CAD build for the part. Positions are in the model's coordinates, mm. Round coordinates to 2 decimals unless told otherwise and drop trailing zeros. Write each loop counter-clockwise with the first axis right and the second up, starting at its lowest first coordinate (ties: lowest second). Pieces come first, ordered by that corner, then holes. Notation, with made-up numbers: (-32.75, -35) - (-11.75, -35) arc R10 cw to (-11.75, -28) - close; hole circle Ø6 at (79, 42.25). An arc over 180 degrees is marked (long way). Put each result on its own line as item: value. Start each with the question number.
Item 1: Mould opens along X. For faces 1 (the flat face through (1, 6, 3)), 2 (the flat face through (4, 6, 1)), 3 (the cylindrical face through (2, 4.3, 1.5)), 4 (the flat face through (-2.5, 6, 1)) say: released by +X, released by -X, zero draft, split by the parting line, or undercut.
Item 2: Drill centre lines: line 1 (Y direction, x = 2, z = 1.75) (3 decimals); line 2 (X direction, y = 10.7, z = 0.8) (3 decimals); line 3 (Y direction, x = 1.75, z = 0.9). Where is each one in solid material? Low to high. Write a range as from..to.
Item 3: Cut at C-C (z = 1.8). Give the cut face in (x, y) (3 decimals).
Item 4: Cut at A-A (x = 2). Give the cut face in (y, z) (3 decimals).
Item 5: Cut at B-B (y = 1.3). Give the cut face in (x, z) (3 decimals), and give its area (3 significant figures).
Item 6: Cut at D-D (y = 3.5). Give the cut face in (x, z), and give its area (3 significant figures).
Autodesk Inventor part; units mm, degrees
ref_plane "YZ Plane" through (0, 0, 0) normal (1, 0, 0) x (0, 1, 0)
ref_plane "XZ Plane" through (0, 0, 0) normal (0, 1, 0) x (-1, 0, 0)
ref_plane "XY Plane" through (0, 0, 0) normal (0, 0, 1) x (1, 0, 0)
sketch "스케치1" plane through (0, 0, 0) normal (0, 0, 1) x (1, 0, 0)
  line L0 (0, 0) -> (4, 0)
  line L1 (4, 0) -> (4, 12)
  line L2 (4, 12) -> (0, 12)
  line L3 (0, 12) -> (0, 0)
  dimension "d0" = 4
  dimension "d1" = 12
extrude "돌출1" add sketch "스케치1" along normal blind 3
sketch "스케치2" plane through (0, 0, 3) normal (0, 0, 1) x (1, 0, 0)
  line L0 (4, 12) -> (0, 12) construction
  line L1 (2, 12) -> (2, 0) construction
  line L2 (0, 0) -> (4, 0) construction
  line L3 (4, 0) -> (4, 12)
  line L4 (0, 12) -> (0, 0)
  point P0 (2, 7.7)
  point P1 (2, 3.5)
  point P2 (2, 1.3)
  point P3 (2, 10.7)
  dimension "d9" = 4.3
  dimension "d45" = 1.3
  dimension "d51" = 4.2
  dimension "d52" = 2.2
  dimension "d55" = 1.3
hole "구멍2" at (2, 3.5, 3) direction (0, 0, -1) diameter 1.6 end through all
hole "구멍3" at (2, 1.3, 3) at (2, 10.7, 3) direction (0, 0, -1) diameter 0.63 end through all
sketch "스케치4" plane through (0, 0, 0) normal (-1, 0, 0) x (0, 0, 1)
  line L0 (0, 12) -> (0, 0)
  line L1 (0, 0) -> (3, 0)
  line L2 (3, 12) -> (3, 0)
  line L3 (0, 12) -> (3, 12)
extrude "돌출4" add sketch "스케치4" along normal blind 2.5
equation "\"G23_M\" = 0.67"
equation "\"G23_F\" = 0.65"
properties part number "_3D 인쇄"
Output values:
1. face 1: zero draft
1. face 2: released by +X
1. face 3: undercut
1. face 4: released by -X
2. line 1: 0..0.985, 1.615..2.7, 4.3..10.385, 11.015..12
2. line 2: -2.5..1.685, 2.315..4
2. line 3: 0..1.11, 1.49..2.74, 4.26..10.51, 10.89..12
3. outline: (-2.5, 0) - (4, 0) - (4, 12) - (-2.5, 12) - close; hole circle Ø1.6 at (2, 3.5); hole circle Ø0.63 at (2, 1.3); hole circle Ø0.63 at (2, 10.7)
4. outline: (0, 0) - (0.985, 0) - (0.985, 3) - (0, 3) - close; (1.615, 0) - (2.7, 0) - (2.7, 3) - (1.615, 3) - close; (4.3, 0) - (10.385, 0) - (10.385, 3) - (4.3, 3) - close; (11.015, 0) - (12, 0) - (12, 3) - (11.015, 3) - close
5. outline: (-2.5, 0) - (1.685, 0) - (1.685, 3) - (-2.5, 3) - close; (2.315, 0) - (4, 0) - (4, 3) - (2.315, 3) - close
5. area: 17.6 mm2
6. outline: (-2.5, 0) - (1.2, 0) - (1.2, 3) - (-2.5, 3) - close; (2.8, 0) - (4, 0) - (4, 3) - (2.8, 3) - close
6. area: 14.7 mm2
